Model file for the job. Use its own axes, mm. A direction names the side the tool comes from. Coordinates: 2 decimals unless noted, no trailing zeros. Write each loop counter-clockwise with the first axis right and the second up, starting at its lowest first coordinate (ties: lowest second). Pieces come first, ordered by that corner, then holes. Notation, with made-up numbers: M 78.5,53 L 123.5,53 A14 ccw 123.5,77 Z; hole C -4,32 d7. An arc over 180 degrees is marked long. Put each result on its own line as item: value. Start each with the question number.
Q1. Cut at D-D (x = -6). Write the cut outline in (y, z), then the cut area to 3 significant figures.
Q2. Cut at B-B (z = 0). Write the cut outline in (x, y).
Q3. Which spindle directions (+Z, -Z, +X, -X, +Y, -Y) get a long thin tool onto all of the face, cutting with end or side? Do faces 1 (the flat face through (-9, 3.5, 9)), 2 (the cylindrical face through (18.412, 1.014, 10.382)), 3 (the flat face through (-20, 1, 2)). Say none if no direction does.
Q4. Drill centre lines: line 1 along Y through (x, z) = (-11, 17.5); line 2 along Z through (x, y) = (4.5, 7); line 3 along X through (y, z) = (2.5, 7.5). Where is each one in solid material? Low to high.
Q5. Cut at A-A (x = 0). Write the cut outline in (y, z), then the cut area to 3 significant figures.
Q6. Cut at C-C (y = 4.25). Write the cut outline in (x, z), then the cut area to 3 significant figures.
Q7. Pull direction Z, two halves, no side cores. Call faces 4 (the cylindrical face through (-23.04, 0.99, 2.33)), 5 (the flat face through (-10, 2, -11)), 6 (the cylindrical face through (23.48, 0.99, 0.99)): pulls with the +Z half, pulls with the -Z half, needs draft (parallel to the pull), parting line crosses it, or undercut.
Q8. Drop flat-ended pins along their axis: pin 1 (1 mm diameter, centred on x = 9, y = 1, fed in from -Z); pin 2 (1.6 mm diameter, centred on x = -20, y = 0.5, fed in from +Z); pin 3 (0.6 mm diameter, centred on x = -20, y = 1, fed in from -Z). Give the stop position or say it passes through.
```python
from build123d import *

# Parameters (mm, degrees)
SKETCH_1_R          = 23.5
SKETCH_1_R_2        = 10
SKETCH_1_R_3        = 1
EXTRUDE_1_DEPTH     = 2
SKETCH_2_R          = 12.5
SKETCH_2_R_2        = 10
EXTRUDE_2_DEPTH     = 5.5
SKETCH_3_R          = 13.5
SKETCH_3_R_2        = 12.5
EXTRUDE_3_DEPTH     = 1.5
SKETCH_4_W          = 7.756986748
SKETCH_4_H          = 4
CUT_EXTRUDE_1_DEPTH = 10
FILLET_1_R          = 1
HOLE_WIZARD_M4_1_D  = 3.3


with BuildPart() as part:
    # 草图1 → 凸台-拉伸1 (new body)
    with BuildSketch(Plane(origin=(0, 0, 0), x_dir=(1, 0, 0), z_dir=(0, 1, 0))):
        with Locations(Location((0, 0, 0), (0, 0, 270))):
            Circle(SKETCH_1_R)
        with Locations(Location((0, 0, 0), (0, 0, 270))):
            Circle(SKETCH_1_R_2, mode=Mode.SUBTRACT)
        with Locations(Location((0, 19.5, 0), (0, 0, 270))):
            Circle(SKETCH_1_R_3, mode=Mode.SUBTRACT)
        with Locations(Location((16.887495374, 9.75, 0), (0, 0, 270))):
            Circle(SKETCH_1_R_3, mode=Mode.SUBTRACT)
        with Locations(Location((16.887495374, -9.75, 0), (0, 0, 270))):
            Circle(SKETCH_1_R_3, mode=Mode.SUBTRACT)
        with Locations(Location((0, -19.5, 0), (0, 0, 270))):
            Circle(SKETCH_1_R_3, mode=Mode.SUBTRACT)
        with Locations(Location((-16.887495374, -9.75, 0), (0, 0, 270))):
            Circle(SKETCH_1_R_3, mode=Mode.SUBTRACT)
        with Locations(Location((-16.887495374, 9.75, 0), (0, 0, 270))):
            Circle(SKETCH_1_R_3, mode=Mode.SUBTRACT)
    extrude(amount=EXTRUDE_1_DEPTH)

    # 草图2 → 凸台-拉伸2 (add)
    with BuildSketch(Plane(origin=(0, 2, 0), x_dir=(1, 0, 0), z_dir=(0, 1, 0))):
        with Locations(Location((0, 0, 0), (0, 0, 270))):
            Circle(SKETCH_2_R)
        with Locations(Location((0, 0, 0), (0, 0, 270))):
            Circle(SKETCH_2_R_2, mode=Mode.SUBTRACT)
    extrude(amount=EXTRUDE_2_DEPTH)

    # 草图3 → 凸台-拉伸3 (add)
    with BuildSketch(Plane(origin=(0, 2, 0), x_dir=(1, 0, 0), z_dir=(0, 1, 0))):
        with Locations(Location((0, 0, 0), (0, 0, 270))):
            Circle(SKETCH_3_R)
        with Locations(Location((0, 0, 0), (0, 0, 270))):
            Circle(SKETCH_3_R_2, mode=Mode.SUBTRACT)
    extrude(amount=EXTRUDE_3_DEPTH)

    # 草图4 → 切除-拉伸1 (cut)
    with BuildSketch(Plane.XZ):
        with Locations((-20.378493374, 0)):
            Rectangle(SKETCH_4_W, SKETCH_4_H)
    extrude(amount=-CUT_EXTRUDE_1_DEPTH, mode=Mode.SUBTRACT)

    # 圆角1
    fillet_1_edges = [part.edges().sort_by_distance(p)[0] for p in [
        (-23.414738948, 1, -2),
        (-23.414738948, 1, 2),
        (-16.5, 1, 2),
        (-16.5, 1, -2),
    ]]
    fillet(fillet_1_edges, radius=FILLET_1_R)

    # M4 螺纹孔1 (through all)
    with Locations(Plane(origin=(0, 0, 0), x_dir=(-1, 0, 0), z_dir=(0, -1, 0))):
        with Locations((0, 19.5), (-16.887495374, 9.75), (-16.887495374, -9.75), (0, -19.5), (16.887495374, -9.75), (16.887495374, 9.75)):
            Hole(HOLE_WIZARD_M4_1_D / 2)


solid = part.part
```
Computed values:
1. outline: M 0,-22.72 L 2,-22.72 L 2,-12.09 L 3.5,-12.09 L 3.5,-10.97 L 7.5,-10.97 L 7.5,-8 L 0,-8 Z; M 0,8 L 7.5,8 L 7.5,10.97 L 3.5,10.97 L 3.5,12.09 L 2,12.09 L 2,22.72 L 0,22.72 Z
1. area: 94.9 mm2
2. outline: M -16.5,0 L -10,0 L -10,7.5 L -12.5,7.5 L -12.5,3.5 L -13.5,3.5 L -13.5,2 L -16.5,2 Z; M 10,0 L 23.5,0 L 23.5,2 L 13.5,2 L 13.5,3.5 L 12.5,3.5 L 12.5,7.5 L 10,7.5 Z
3. face 1: +Y
3. face 2: +Y, -Y
3. face 3: -X, +Y, -Y
4. line 1: 0 to 2
4. line 2: -11.66 to -8.93, 8.93 to 11.66
4. line 3: -11.22 to -6.61, 6.61 to 11.22
5. outline: M 0,-23.5 L 2,-23.5 L 2,-21.15 L 0,-21.15 Z; M 0,-17.85 L 2,-17.85 L 2,-13.5 L 3.5,-13.5 L 3.5,-12.5 L 7.5,-12.5 L 7.5,-10 L 0,-10 Z; M 0,10 L 7.5,10 L 7.5,12.5 L 3.5,12.5 L 3.5,13.5 L 2,13.5 L 2,17.85 L 0,17.85 Z; M 0,21.15 L 2,21.15 L 2,23.5 L 0,23.5 Z
5. area: 71.3 mm2
6. outline: C 0,0 d25; hole C 0,0 d20
6. area: 177 mm2
7. face 4: undercut
7. face 5: needs draft
7. face 6: parting line crosses it
8. pin 1: z = -21.91
8. pin 2: z = 13.55
8. pin 3: z = -12.81
